from build123d import *

# Parameters (mm, degrees)
ESBO_O1_R                = 6
ESBO_O1_R_2              = 4.1
RESSALTO_EXTRUS_O1_DEPTH = 2
ESBO_O2_W                = 40
ESBO_O2_H                = 4
RESSALTO_EXTRUS_O2_DEPTH = 6
CHANFRO3_SIZE            = 10
CHANFRO4_SIZE            = 10
CHANFRO5_SIZE            = 10
ESBO_O6_R                = 2.6
CORTE_EXTRUS_O2_DEPTH    = 39.574603044
ESBO_O7_R                = 5.25
CORTE_EXTRUS_O6_DEPTH    = 39.574603044
FILETE1_R                = 3


with BuildPart() as part:
    # Esboço1 → Ressalto-extrusão1 (new, symmetric)
    # profile 1 of 3: a face of its own
    with BuildSketch(Plane(origin=(0, 0, 0), x_dir=(1, 0, 0), z_dir=(0, 1, 0))):
        Polygon((20, 18), (-20, 18), (-20, 14), (-6, 14), (6, 14), (20, 14), align=None)
    # profile 2 of 3: a face of its own
    with BuildSketch(Plane(origin=(0, 0, 0), x_dir=(1, 0, 0), z_dir=(0, 1, 0))):
        with BuildLine():
            Line((6, 14), (-6, 14))
            Line((-6, 14), (-6, -12))
            ThreePointArc((-6, -12), (0, -6), (6, -12))
            Line((6, -12), (6, 14))
        make_face()
    # profile 3 of 3: a face of its own
    with BuildSketch(Plane(origin=(0, 0, 0), x_dir=(1, 0, 0), z_dir=(0, 1, 0))):
        with Locations((0, -12)):
            Circle(ESBO_O1_R)
        with Locations(Location((0, -12, 0), (0, 0, 270))):
            Circle(ESBO_O1_R_2, mode=Mode.SUBTRACT)
    extrude(amount=RESSALTO_EXTRUS_O1_DEPTH, both=True)

    # Esboço2 → Ressalto-extrusão2 (add)
    with BuildSketch(Plane(origin=(0, 2, 0), x_dir=(1, 0, 0), z_dir=(0, 1, 0))):
        with Locations((0, 16)):
            Rectangle(ESBO_O2_W, ESBO_O2_H)
    extrude(amount=RESSALTO_EXTRUS_O2_DEPTH)

    # Chanfro3
    chanfro3_edges = [part.edges().sort_by_distance(p)[0] for p in [
        (6, 0, -14),
    ]]
    chamfer(chanfro3_edges, length=CHANFRO3_SIZE)

    # Chanfro4
    chanfro4_edges = [part.edges().sort_by_distance(p)[0] for p in [
        (-6, 0, -14),
    ]]
    chamfer(chanfro4_edges, length=CHANFRO4_SIZE)

    # Chanfro5
    # the kernel refuses this chamfer: 10 mm, written as the material it adds along each edge
    with BuildSketch(Plane(origin=(-41.71682988, 2, -14), x_dir=(0, 0.9996219169112968, -0.027495876610586317), z_dir=(1, 0, 0))) as chanfro5_piece_1_section:
        Polygon((CHANFRO5_SIZE * 0.999621916911, CHANFRO5_SIZE * 0.0274958766106), (-CHANFRO5_SIZE * 0.0274958766106, CHANFRO5_SIZE * 0.999621916911), (0, 0), align=None)
    chanfro5_piece_1 = extrude(amount=83.433659759, mode=Mode.PRIVATE)
    chanfro5_piece_1 = split(chanfro5_piece_1, bisect_by=Plane(origin=(-11.43705518, 4.703831668, -9.43705518), z_dir=(0.7071067811865475, 0, -0.7071067811865476)), keep=Keep.TOP, mode=Mode.PRIVATE)
    chanfro5_piece_1 = split(chanfro5_piece_1, bisect_by=Plane(origin=(-9.624703453, 8, -11.249406907), z_dir=(0, -1, 0)), keep=Keep.TOP, mode=Mode.PRIVATE)
    chanfro5_piece_1 = split(chanfro5_piece_1, bisect_by=Plane(origin=(-6, 4.703831668, -11.249406907), z_dir=(-1, 0, 0)), keep=Keep.TOP, mode=Mode.PRIVATE)
    add(chanfro5_piece_1)
    with BuildSketch(Plane(origin=(-41.71682988, 2, -14), x_dir=(0, 0.9996219169112968, -0.027495876610586317), z_dir=(1, 0, 0))) as chanfro5_piece_2_section:
        Polygon((CHANFRO5_SIZE * 0.999621916911, CHANFRO5_SIZE * 0.0274958766106), (-CHANFRO5_SIZE * 0.0274958766106, CHANFRO5_SIZE * 0.999621916911), (0, 0), align=None)
    chanfro5_piece_2 = extrude(amount=83.433659759, mode=Mode.PRIVATE)
    chanfro5_piece_2 = split(chanfro5_piece_2, bisect_by=Plane(origin=(-6.125087245, 4.433681659, -4.125087245), z_dir=(0.7071067811865475, 0, -0.7071067811865476)), keep=Keep.TOP, mode=Mode.PRIVATE)
    chanfro5_piece_2 = split(chanfro5_piece_2, bisect_by=Plane(origin=(6.125087245, 4.433681659, -4.125087245), z_dir=(-0.7071067811865477, 0, -0.7071067811865474)), keep=Keep.TOP, mode=Mode.PRIVATE)
    chanfro5_piece_2 = split(chanfro5_piece_2, bisect_by=Plane(origin=(0, 8, -10.250174491), z_dir=(0, -1, 0)), keep=Keep.TOP, mode=Mode.PRIVATE)
    chanfro5_piece_2 = split(chanfro5_piece_2, bisect_by=Plane(origin=(6, 4.433681659, -10.250174491), z_dir=(-1, 0, 0)), keep=Keep.TOP, mode=Mode.PRIVATE)
    chanfro5_piece_2 = split(chanfro5_piece_2, bisect_by=Plane(origin=(-6, 4.433681659, -10.250174491), z_dir=(1, 0, 0)), keep=Keep.TOP, mode=Mode.PRIVATE)
    add(chanfro5_piece_2)
    with BuildSketch(Plane(origin=(-41.71682988, 2, -14), x_dir=(0, 0.9996219169112968, -0.027495876610586317), z_dir=(1, 0, 0))) as chanfro5_piece_3_section:
        Polygon((CHANFRO5_SIZE * 0.999621916911, CHANFRO5_SIZE * 0.0274958766106), (-CHANFRO5_SIZE * 0.0274958766106, CHANFRO5_SIZE * 0.999621916911), (0, 0), align=None)
    chanfro5_piece_3 = extrude(amount=83.433659759, mode=Mode.PRIVATE)
    chanfro5_piece_3 = split(chanfro5_piece_3, bisect_by=Plane(origin=(11.43705518, 4.703831668, -9.43705518), z_dir=(-0.7071067811865477, 0, -0.7071067811865474)), keep=Keep.TOP, mode=Mode.PRIVATE)
    chanfro5_piece_3 = split(chanfro5_piece_3, bisect_by=Plane(origin=(9.624703453, 8, -11.249406907), z_dir=(0, -1, 0)), keep=Keep.TOP, mode=Mode.PRIVATE)
    chanfro5_piece_3 = split(chanfro5_piece_3, bisect_by=Plane(origin=(6, 4.703831668, -11.249406907), z_dir=(1, 0, 0)), keep=Keep.TOP, mode=Mode.PRIVATE)
    add(chanfro5_piece_3)

    # Esboço6 → Corte-extrusão2 (cut, symmetric)
    with BuildSketch(Plane.XY.offset(-14)):
        with Locations((-15, 3)):
            Circle(ESBO_O6_R)
    corte_extrus_o2 = extrude(amount=CORTE_EXTRUS_O2_DEPTH, both=True, mode=Mode.SUBTRACT)

    # Esboço7 → Corte-extrusão6 (cut, through all)
    with BuildSketch(Plane.XY.offset(-14)):
        with Locations((-15, 3)):
            Circle(ESBO_O7_R)
    corte_extrus_o6 = extrude(amount=CORTE_EXTRUS_O6_DEPTH, mode=Mode.SUBTRACT)

    # Espelhar2: Corte-extrusão2, Corte-extrusão6 across plane
    add(corte_extrus_o2.mirror(Plane(origin=(0, 0, 0), x_dir=(0, 0, 1), z_dir=(1, 0, 0))), mode=Mode.SUBTRACT)
    add(corte_extrus_o6.mirror(Plane(origin=(0, 0, 0), x_dir=(0, 0, 1), z_dir=(1, 0, 0))), mode=Mode.SUBTRACT)

    # Filete1
    filete1_edges = [part.edges().sort_by_distance(p)[0] for p in [
        (20, -2, -16),
        (-20, -2, -16),
        (-20, 8, -16),
        (20, 8, -16),
    ]]
    fillet(filete1_edges, radius=FILETE1_R)


solid = part.part
Model file for the job. Use its own axes, mm. A direction names the side the tool comes from. Coordinates: 2 decimals unless noted, no trailing zeros. Order: outer loops, then holes, each group sorted by start corner. A loop starts at its lowest first (then second) coordinate and runs counter-clockwise, first axis right, second up. Notation, with made-up numbers: M -16.75,34.5 L 34.25,34.5 A13 ccw 34.25,59.5 Z; hole C -27,22.5 d2. An arc over 180 degrees is marked long. Return JSON: item names as keys, results as strings.
1. Tool access for faces 4 (the face through (-6, 0, 4)), 5 (the face through (9.75, 2.91, -11.61)), 6 (the face through (6, 0, 4)), 7 (the face through (0, 2, 4)), 8 (the face through (-9.75, 2.91, -11.61)): list every direction of +Z, -Z, +X, -X, +Y, -Y with a clear straight run to the whole face (end or side of a thin tool).
Ans:
{"face 4": "+Z, -X, +Y, -Y", "face 5": "+Z, +X", "face 6": "+Z, +X, +Y, -Y", "face 7": "+Z, +X, -X, +Y", "face 8": "+Z, -X"}
2. Saw through at C-C (x = -15). Give the cut face in (y, z).
Ans:
{"outline": "M -2,-18 L 0.4,-18 L 0.4,-14 L -2,-14 Z; M 5.6,-18 L 8,-18 L 8,-14 L 5.6,-14 Z"}
3. Saw through at A-A (x = 0). Give the cut face in (y, z), and give its area (3 significant figures).
Ans:
{"outline": "M -2,-18 L 8,-18 L 8,-10 L 2,-4 L 2,7.9 L -2,7.9 Z; M -2,16.1 L 2,16.1 L 2,18 L -2,18 Z", "area": "177 mm^2"}
4. Saw through at D-D (y = 7.25). Give the cut face in (x, z).
Ans:
{"outline": "M -18.98,-18 L 18.98,-18 L 18.98,-14 L 11.92,-14 L 11.92,-9.92 L 11.25,-9.25 L -11.25,-9.25 L -11.92,-9.92 L -11.92,-14 L -18.98,-14 Z"}
5. Pull direction Y, two halves, no side cores. Call faces 1 (the face through (20, 3, -16)), 2 (the face through (19.1, -1.14, -16.03)), 3 (the face through (12.5, 1.8, -14)): +Y half, -Y half, draft (parallel to the pull), parting line (faces both ways), or undercut.
Ans:
{"face 1": "draft", "face 2": "-Y half", "face 3": "undercut"}
6. Drill centre lines: probe 1 along X at (y, z) = (3, -16.7); probe 2 along Y at (x, z) = (15, -15); probe 3 along Y at (x, z) = (-4.5, 2.5). Where is each one in solid material? Low to high.
Ans:
{"probe 1": "-20 to -17.6, -12.4 to 12.4, 17.6 to 20", "probe 2": "-2 to 0.4, 5.6 to 8", "probe 3": "-2 to 2"}
7. Flat gauge pins, fed straight in: pin 1 (3 mm diameter, centred on y = -0.5, z = 3, fed in from +X); pin 2 (1 mm diameter, centred on x = -8, y = 1.5, fed in from +Z); pin 3 (2 mm diameter, centred on y = 1, z = 1, fed in from -X). Where does each tip first touch, or does it go through?
Ans:
{"pin 1": "x = 6", "pin 2": "z = -5.5", "pin 3": "x = -6"}
8. Saw through at B-B (z = 14.5). Give the cut face in (x, y).
Ans:
{"outline": "M -5.45,-2 L -3.25,-2 L -3.25,2 L -5.45,2 Z; M 3.25,-2 L 5.45,-2 L 5.45,2 L 3.25,2 Z"}
